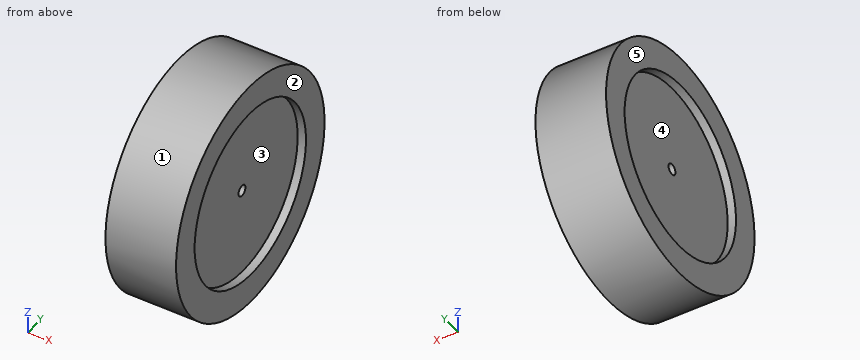
from build123d import *

# Parameters (mm, degrees)
ESQUISSE1_R             = 28
BOSS_EXTRU_1_DEPTH      = 17
ESQUISSE2_R             = 1.3
ENL_V_MAT_EXTRU_1_DEPTH = 17
ESQUISSE3_R             = 21
ENL_V_MAT_EXTRU_2_DEPTH = 2


with BuildPart() as part:
    # Esquisse1 → Boss.-Extru.1 (new body)
    with BuildSketch(Plane(origin=(0, 0, 0), x_dir=(0, 0, -1), z_dir=(1, 0, 0))):
        Circle(ESQUISSE1_R)
    extrude(amount=BOSS_EXTRU_1_DEPTH)

    # Esquisse2 → Enlèv. mat.-Extru.1 (cut)
    with BuildSketch(Plane(origin=(17, 0, 0), x_dir=(0, 0, -1), z_dir=(1, 0, 0))):
        Circle(ESQUISSE2_R)
    extrude(amount=-ENL_V_MAT_EXTRU_1_DEPTH, mode=Mode.SUBTRACT)

    # Esquisse3 → Enlèv. mat.-Extru.2 (cut)
    with BuildSketch(Plane(origin=(17, 0, 0), x_dir=(0, 0, -1), z_dir=(1, 0, 0))):
        Circle(ESQUISSE3_R)
    enl_v_mat_extru_2 = extrude(amount=-ENL_V_MAT_EXTRU_2_DEPTH, mode=Mode.SUBTRACT)

    # Symétrie1: Enlèv. mat.-Extru.2 across plane
    add(enl_v_mat_extru_2.mirror(Plane(origin=(8.5, 0, 0), x_dir=(0, 0, 1), z_dir=(1, 0, 0))), mode=Mode.SUBTRACT)


solid = part.part
Can you work these out from the model? Positions are in its coordinate system, mm. Face numbers are marked on the shaded views. A direction names the side the tool comes from. Give positions to 0.01 mm unless a question says otherwise; leave off trailing zeros. Order: outer loops, then holes, each group sorted by start corner. A loop starts at its lowest first (then second) coordinate and runs counter-clockwise, first axis right, second up. Notation, with made-up numbers: M 38.25,-15 L 78.25,-15 A25 ccw 78.25,10 Z; hole C -29.75,25 d4. An arc over 180 degrees is marked long. One line per question, with ' | ' between items.
Item 1: We'd pull the mould along Z, two halves only. Please class the marked faces 1, 2 and 3: released by +Z, released by -Z, zero draft, split by the parting line, or undercut.
Answer block:
face 1: split by the parting line | face 2: zero draft | face 3: undercut
Item 2: For the marked faces 4 and 5, which set-ups out of +Z, -Z, +X, -X, +Y, -Y let a thin tool reach every point of the face, with its end or its side?
Answer block:
face 4: -X | face 5: +Z, -Z, -X, +Y, -Y
Item 3: Suppose I cut it at C-C, the plane z = 8.5. Write out the boundary of the cut face in (x, y).
Answer block:
outline: M 0,-26.68 L 17,-26.68 L 17,-19.2 L 15,-19.2 L 15,19.2 L 17,19.2 L 17,26.68 L 0,26.68 L 0,19.2 L 2,19.2 L 2,-19.2 L 0,-19.2 Z
Item 4: Please list where these lines run through material, in increasing order: L1, parallel to Y at x = 11.75, z = 0; L2, parallel to Y at x = 16.3, z = 0; L3, parallel to X at y = 18, z = 4.
Answer block:
L1: y = -28 to -1.3, 1.3 to 28 | L2: y = -28 to -21, 21 to 28 | L3: x = 2 to 15
Item 5: I'm going to push flat-ended pins straight in: pin 1 Ø2 at (y, z) = (0, 0) entering from +X; pin 2 Ø3 at (x, z) = (7.5, -17) entering from +Y; pin 3 Ø5 at (y, z) = (2, 2.5) entering from +X; pin 4 Ø3 at (x, z) = (15.5, 12) entering from +Y. Where does each tip first touch, or does it pass through?
Answer block:
pin 1: passes through | pin 2: stops at y = 23.32 | pin 3: stops at x = 15 | pin 4: stops at y = 25.96
Item 6: Suppose I cut it at A-A, the plane z = 0. Write out the boundary of the cut face in (x, y), then the cut area to 3 significant figures.
Answer block:
outline: M 0,-28 L 17,-28 L 17,-21 L 15,-21 L 15,-1.3 L 2,-1.3 L 2,-21 L 0,-21 Z; M 0,21 L 2,21 L 2,1.3 L 15,1.3 L 15,21 L 17,21 L 17,28 L 0,28 Z | area: 750 mm2
Item 7: Suppose I cut it at D-D, the plane x = 6.5. Write out the boundary of the cut face in (y, z), then the cut area to 3 significant figures.
Answer block:
outline: C 0,0 d56; hole C 0,0 d2.6 | area: 2,460 mm2
